from build123d import *

# Parameters (mm, degrees)
SKETCH1_W                      = 45
SKETCH1_H                      = 48
BOSS_EXTRUDE1_DEPTH            = 25
SKETCH2_W                      = 22.9
SKETCH2_H                      = 45.9
CUT_EXTRUDE1_DEPTH             = 70.666419457
F_24_0_24_DIAMETER_HOLE1_D     = 24
F_24_0_24_DIAMETER_HOLE1_DEPTH = 25
F_3_2_3_2_DIAMETER_HOLE1_D     = 3.2
F_3_2_3_2_DIAMETER_HOLE1_DEPTH = 25
F_3_2_3_2_DIAMETER_HOLE2_D     = 3.2
FILLET1_R                      = 2
FILLET2_R                      = 3
F_3_0_3_DIAMETER_HOLE1_D       = 3


with BuildPart() as part:
    # Sketch1 → Boss-Extrude1 (new body)
    with BuildSketch(Plane(origin=(2.1, 0, 0), x_dir=(0, 0, -1), z_dir=(1, 0, 0))):
        with Locations((0, 24)):
            Rectangle(SKETCH1_W, SKETCH1_H)
    extrude(amount=-BOSS_EXTRUDE1_DEPTH)

    # Sketch2 → Cut-Extrude1 (cut, through all)
    with BuildSketch(Plane(origin=(0, 0, -22.5), x_dir=(-1, 0, 0), z_dir=(0, 0, -1))):
        with Locations((11.45, 25.05)):
            Rectangle(SKETCH2_W, SKETCH2_H)
    extrude(amount=-CUT_EXTRUDE1_DEPTH, mode=Mode.SUBTRACT)

    # Ø24.0 (24) Diameter Hole1
    with Locations(Plane(origin=(2.1, 0, 0), x_dir=(0, 0, -1), z_dir=(1, 0, 0))):
        with Locations((0, 25)):
            Hole(F_24_0_24_DIAMETER_HOLE1_D / 2, depth=F_24_0_24_DIAMETER_HOLE1_DEPTH)

    # Ø3.2 (3.2) Diameter Hole1
    with Locations(Plane(origin=(2.1, 0, 0), x_dir=(0, 0, -1), z_dir=(1, 0, 0))):
        with Locations((15.5, 9.5), (-15.5, 40.5), (15.5, 40.5), (-15.5, 9.5)):
            Hole(F_3_2_3_2_DIAMETER_HOLE1_D / 2, depth=F_3_2_3_2_DIAMETER_HOLE1_DEPTH)

    # Ø3.2 (3.2) Diameter Hole2 (through all)
    with Locations(Plane(origin=(0, 2.1, 0), x_dir=(1, 0, 0), z_dir=(0, 1, 0))):
        with Locations((-10.4, 12.5), (-10.4, -12.5)):
            Hole(F_3_2_3_2_DIAMETER_HOLE2_D / 2)

    # Fillet1
    fillet1_edges = [part.edges().sort_by_distance(p)[0] for p in [
        (2.1, 0, 0),
    ]]
    fillet(fillet1_edges, radius=FILLET1_R)

    # Fillet2
    fillet2_edges = [part.edges().sort_by_distance(p)[0] for p in [
        (-22.9, 1.05, 22.5),
        (1.05, 48, -22.5),
        (1.05, 48, 22.5),
        (-22.9, 1.05, -22.5),
    ]]
    fillet(fillet2_edges, radius=FILLET2_R)

    # Ø3.0 (3) Diameter Hole1 (through all)
    with Locations(Plane(origin=(0, 2.1, 0), x_dir=(1, 0, 0), z_dir=(0, 1, 0))):
        with Locations((-2.10285259, 8.031001386), (-2.10285259, -7.968998614), (-17.10285259, 8.031001386), (-17.10285259, -7.968998614)):
            Hole(F_3_0_3_DIAMETER_HOLE1_D / 2)


solid = part.part
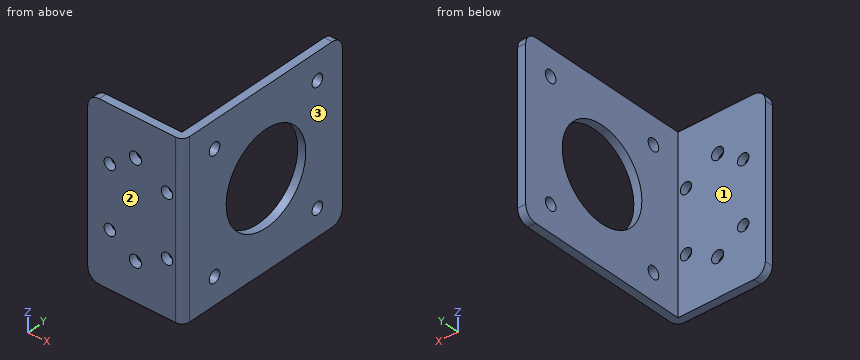
The listing builds one solid part. Answer for the finished solid, in the listing's coordinates (mm). Face numbers are marked on the shaded views. Round coordinates to 2 decimals unless told otherwise and drop trailing zeros. Write each loop counter-clockwise with the first axis right and the second up, starting at its lowest first coordinate (ties: lowest second). Pieces come first, ordered by that corner, then holes. Notation, with made-up numbers: M 44,43 L 102,43 A22 ccw 102,72 Z; hole C 86.5,16.25 d2. An arc over 180 degrees is marked long. Write each question's results on one line, items separated by ' | '. Start each with the question number.
Item 1: For a pull along Y with two mould halves and no side action, classify the marked faces 1, 2 and 3 as pulls with the +Y half, pulls with the -Y half, needs draft (parallel to the pull), parting line crosses it, or undercut.
Item 2: A cutting plane is placed at C-C on y = 9.5. Write down the section's boundary in (x, z).
Item 3: A cutting plane is placed at A-A on x = -10.4. Write down the section's boundary in (y, z), and give its area (3 significant figures).
Item 4: A cutting plane is placed at D-D on z = 1. Write down the section's boundary in (x, y), and give its area (3 significant figures).
Item 5: Straight lines are drawn through the part: L1, parallel to Y at x = 1.55, z = -15.5; L2, parallel to Y at x = 0.95, z = 15.5; L3, parallel to Y at x = -18.75, z = 14.5. For each, find the intervals that lie inside material, in ascending order. Write a range as [from, to].
Item 6: Flat-ended cylindrical pins translate along their axes: pin 1 Ø8 at (x, y) = (-6.5, 10.5) entering from -Z; pin 2 Ø8 at (x, z) = (-20, -5) entering from +Y; pin 3 Ø3 at (y, z) = (20, 13) entering from -X. Find the tip coordinate at first contact, or state that the pin passes through.
Item 7: A cutting plane is placed at B-B on z = 15.5. Write down the section's boundary in (x, y).
Check sheet entries:
1) face 1: pulls with the +Y half | face 2: pulls with the -Y half | face 3: needs draft
2) outline: M 0,-22.5 L 2.1,-22.5 L 2.1,-17.1 L 0,-17.1 Z; M 0,-13.9 L 2.1,-13.9 L 2.1,13.9 L 0,13.9 Z; M 0,17.1 L 2.1,17.1 L 2.1,22.5 L 0,22.5 Z
3) outline: M 0,-22.5 L 2.1,-22.5 L 2.1,-14.1 L 0,-14.1 Z; M 0,-10.9 L 2.1,-10.9 L 2.1,10.9 L 0,10.9 Z; M 0,14.1 L 2.1,14.1 L 2.1,22.5 L 0,22.5 Z | area: 81.1 mm²
4) outline: M -22.9,0 L 0.1,0 A2 ccw 2.1,2 L 2.1,13.04 L 0,13.04 L 0,2.1 L -22.9,2.1 Z; M 0,36.96 L 2.1,36.96 L 2.1,48 L 0,48 Z | area: 97.8 mm²
5) L1: [0.62, 7.9], [11.1, 38.9], [42.1, 48] | L2: [0.19, 7.9], [11.1, 38.9], [42.1, 48] | L3: [0, 2.1]
6) pin 1: through | pin 2: y = 2.1 | pin 3: x = 0
7) outline: M -22.9,0 L 0.1,0 A2 ccw 2.1,2 L 2.1,7.9 L 0,7.9 L 0,2.1 L -22.9,2.1 Z; M 0,11.1 L 2.1,11.1 L 2.1,38.9 L 0,38.9 Z; M 0,42.1 L 2.1,42.1 L 2.1,48 L 0,48 Z
